```python
from build123d import *

# Parameters (mm, degrees)
F0_W     = 711.2
F0_H     = 31.75
F1_DEPTH = 63.5
F2_W     = 58.42
F2_H     = 29.21
F3_DEPTH = 711.201
F4_W     = 457.2
F4_H     = 31.75
F5_DEPTH = 2.54


with BuildPart() as f1:
    # F0 (on Front) → F1 (new body)
    with BuildSketch(Plane.XZ):
        Rectangle(F0_W, F0_H)
    extrude(amount=F1_DEPTH)

    # F2 (on face) → F3 (cut, through all)
    with BuildSketch(Plane.YZ.offset(355.6)):
        with Locations((-31.75, 1.27)):
            Rectangle(F2_W, F2_H)
    extrude(amount=-F3_DEPTH, mode=Mode.SUBTRACT)

    # F4 (on face) → F5 (cut)
    with BuildSketch(Plane.XZ.offset(63.5)):
        Rectangle(F4_W, F4_H)
    extrude(amount=-F5_DEPTH, mode=Mode.SUBTRACT)


solid = f1.part
```
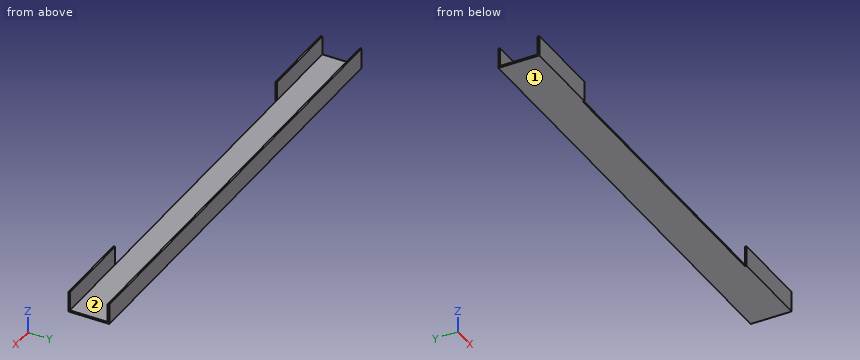
Work out the finished part from the listing and answer in its coordinate system (mm). Face numbers are marked on the shaded views. Coordinates: 2 decimals unless noted, no trailing zeros. Write each loop counter-clockwise with the first axis right and the second up, starting at its lowest first coordinate (ties: lowest second). Pieces come first, ordered by that corner, then holes.
Q1. Find the intervals of material crossed by line 1 (Y direction, x = 297.5, z = 8); line 2 (Y direction, x = -226.5, z = -1); line 3 (Z direction, x = 25.5, y = -24.5) (3 decimals), in increasing order.
Q2. A cutting plane is placed at B-B, the plane x = -292. Give the vertices of the cut face in (y, z) (3 decimals).
Q3. A cutting plane is placed at A-A, the plane z = -6. Give the vertices of the cut face in (x, y).
Q4. A cutting plane is placed at D-D, the plane x = -98.5. Give the vertices of the cut face in (y, z) (3 decimals), then the cut area to 3 significant figures.
Q5. Determine the mould class of the marked faces 1 and 2 for opening direction Y: released by +Y, released by -Y, zero draft, split by the parting line, or undercut.
Q6. A cutting plane is placed at C-C, the plane y = -26. Give the vertices of the cut face in (x, z) (3 decimals).
Q7. Each of these flat-tipped pins is pushed along its axis until it touches: pin 1 Ø3 at (x, y) = (-12.5, -43.5) entering from +Z (3 decimals); pin 2 Ø14.5 at (x, z) = (-45.5, -0.5) entering from -Y; pin 3 Ø2 at (x, z) = (43, -14.5) entering from -Y. Where does it stop, or does it pass through?
Findings below:
1. line 1: y = -63.5 to -60.96, -2.54 to 0
1. line 2: y = -2.54 to 0
1. line 3: z = -15.875 to -13.335
2. outline: (-63.5, -15.875) - (0, -15.875) - (0, 15.875) - (-2.54, 15.875) - (-2.54, -13.335) - (-60.96, -13.335) - (-60.96, 15.875) - (-63.5, 15.875) - close
3. outline: (-355.6, -63.5) - (-228.6, -63.5) - (-228.6, -60.96) - (-355.6, -60.96) - close; (-355.6, -2.54) - (355.6, -2.54) - (355.6, 0) - (-355.6, 0) - close; (228.6, -63.5) - (355.6, -63.5) - (355.6, -60.96) - (228.6, -60.96) - close
4. outline: (-60.96, -15.875) - (0, -15.875) - (0, 15.875) - (-2.54, 15.875) - (-2.54, -13.335) - (-60.96, -13.335) - close
4. area: 229 mm2
5. face 1: zero draft
5. face 2: undercut
6. outline: (-355.6, -15.875) - (355.6, -15.875) - (355.6, -13.335) - (-355.6, -13.335) - close
7. pin 1: stops at z = -13.335
7. pin 2: stops at y = -2.54
7. pin 3: stops at y = -60.96
